```python
from build123d import *

# Parameters (mm, degrees)
EXTRUDE_1_DEPTH = 338
OTHER_START     = -31
OTHER_1_DEPTH   = 5
OTHER_START_2   = -24.7
OTHER_1_2_DEPTH = 20.7
OTHER_START_3   = -1
OTHER_1_3_DEPTH = 5
OTHER_START_4   = 4
OTHER_1_4_DEPTH = 4
OTHER_START_5   = -4
OTHER_1_5_DEPTH = 4
OTHER_START_6   = -26
OTHER_1_6_DEPTH = 18


with BuildPart() as part:
    # Эскиз1 → Бобышка-Вытянуть1 (new body)
    with BuildSketch(Plane.XY):
        with BuildLine():
            Line((0, 0), (0, 30))
            Line((0, 30), (-2.7, 30))
            ThreePointArc((-2.7, 30), (-3.619238816, 29.619238816), (-4, 28.7))
            Line((-4, 28.7), (-4, 8))
            ThreePointArc((-4, 8), (-5.171572875, 5.171572875), (-8, 4))
            Line((-8, 4), (-28.7, 4))
            ThreePointArc((-28.7, 4), (-29.619238816, 3.619238816), (-30, 2.7))
            Line((-30, 2.7), (-30, 0))
            Line((-30, 0), (0, 0))
        make_face()
    extrude(amount=-EXTRUDE_1_DEPTH)

    # Полость1: read off the stored shape, not the designer's step
    # Полость1 outline → Полость1 (cut)
    with BuildSketch(Plane.YZ.offset(OTHER_START)):
        with BuildLine():
            Line((4, -338), (4, -313.3))
            ThreePointArc((4, -313.3), (3.619238816, -312.380761184), (2.7, -312))
            Line((2.7, -312), (0, -312))
            Line((0, -312), (0, -338))
            Line((0, -338), (4, -338))
        make_face()
    extrude(amount=OTHER_1_DEPTH, mode=Mode.SUBTRACT)

    # Other 1 2 outline → Other 1 2 (cut)
    with BuildSketch(Plane.YZ.offset(OTHER_START_2)):
        with BuildLine():
            ThreePointArc((8, -338), (5.171572875, -336.828427125), (4, -334))
            Line((4, -334), (4, -338))
            Line((4, -338), (8, -338))
        make_face()
    extrude(amount=OTHER_1_2_DEPTH, mode=Mode.SUBTRACT)

    # Other 1 3 outline → Other 1 3 (cut)
    with BuildSketch(Plane(origin=(0, 0, 0), x_dir=(1, 0, 0), z_dir=(0, 1, 0)).offset(OTHER_START_3)):
        Polygon((0, 338), (-26, 338), (-26, 312), align=None)
    extrude(amount=OTHER_1_3_DEPTH, mode=Mode.SUBTRACT)

    # Other 1 4 outline → Other 1 4 (cut)
    with BuildSketch(Plane(origin=(0, 0, 0), x_dir=(1, 0, 0), z_dir=(0, 1, 0)).offset(OTHER_START_4)):
        Polygon((-4, 334), (0, 338), (-4, 338), align=None)
    extrude(amount=OTHER_1_4_DEPTH, mode=Mode.SUBTRACT)

    # Other 1 5 outline → Other 1 5 (add)
    with BuildSketch(Plane.YZ.offset(OTHER_START_5)):
        with BuildLine():
            ThreePointArc((4, -334), (5.171572875, -336.828427125), (8, -338))
            Line((8, -338), (8, -311))
            Line((8, -311), (4.000000005, -311))
            Line((4.000000005, -311), (4, -334))
        make_face()
    extrude(amount=OTHER_1_5_DEPTH)

    # Other 1 6 outline → Other 1 6 (add)
    with BuildSketch(Plane.YZ.offset(OTHER_START_6)):
        with BuildLine():
            ThreePointArc((2.7, -312), (3.619238816, -312.380761184), (4, -313.3))
            Line((4, -313.3), (4.000000005, -311))
            Line((4.000000005, -311), (2, -311))
            Line((2, -311), (2, -312.000000001))
            Line((2, -312.000000001), (2.7, -312))
        make_face()
    extrude(amount=OTHER_1_6_DEPTH)

    # Зеркальное отражение1: part across plane


with BuildPart() as part_1:
    add(part.part)
    add(part.part.mirror(Plane(origin=(-2.7, 28.7, 0), x_dir=(1, 0, 0), z_dir=(0, 0, 1))))


solid = part_1.part
```
Input: part model. Units: mm. Frame: model coordinates. A direction names the side the tool comes from. Give positions to 0.01 mm unless a question says otherwise; leave off trailing zeros. Order: outer loops, then holes, each group sorted by start corner. A loop starts at its lowest first (then second) coordinate and runs counter-clockwise, first axis right, second up.
1. Line query: probe 1 along X at (y, z) = (27, 292.5); probe 2 along Y at (x, z) = (-22, -198.5); probe 3 along Z at (x, y) = (-9.5, 3). Output: solid intervals per line, ascending.
Computed:
probe 1: x = -4 to 0
probe 2: y = 0 to 4
probe 3: z = -328.5 to 328.5
2. Draft query along Z for faces 3 (the face through (0, 15, -5)), 4 (the face through (-13, 2, -325)), 5 (the face through (-13, 2, 325)). Return one class per face: released by +Z, released by -Z, zero draft, split by the parting line, or undercut.
Computed:
face 3: zero draft
face 4: released by -Z
face 5: released by +Z
3. Cut plane A-A (z = -141). Return loops of the section in (x, y), and give its area (3 significant figures).
Computed:
outline: (-30, 0) - (0, 0) - (0, 30) - (-2.7, 30) arc R1.3 ccw to (-4, 28.7) - (-4, 8) arc R4 cw to (-8, 4) - (-28.7, 4) arc R1.3 ccw to (-30, 2.7) - close
area: 227 mm2
4. Pin query (flat end, axial travel): pin 1 Ø1.4 at (x, y) = (-28.5, 2) entering from -Z; pin 2 Ø1.5 at (x, z) = (-19.5, -39.5) entering from -Y; pin 3 Ø1.4 at (x, z) = (-25.5, 312.5) entering from +Y; pin 4 Ø6 at (y, z) = (12.5, 222.5) entering from -X. Return the tip coordinate at first contact, or that it passes through.
Computed:
pin 1: stops at z = -312
pin 2: stops at y = 0
pin 3: stops at y = 4
pin 4: stops at x = -4
5. Cut plane B-B (x = -13.5). Return loops of the section in (y, z), and give its area (3 significant figures).
Computed:
outline: (0, -324.5) - (4, -324.5) - (4, 324.5) - (0, 324.5) - close
area: 2,600 mm2
6. Cut plane C-C (y = 19.75). Return loops of the section in (x, z).
Computed:
outline: (-4, -338) - (0, -338) - (0, 338) - (-4, 338) - close
7. Set-up query: faces 1 (the face through (-4, 18, -5)), 2 (the face through (-15, 0, -5)). Return all of +Z, -Z, +X, -X, +Y, -Y with unobstructed straight access to the full face (end or side cutting, diameter ignored); none if empty.
Computed:
face 1: +Z, -Z, -X, +Y
face 2: +Z, -Z, +X, -X, -Y
